Model file for the job. Use its own axes, mm. Coordinates: 2 decimals unless noted, no trailing zeros. Write each loop counter-clockwise with the first axis right and the second up, starting at its lowest first coordinate (ties: lowest second). Pieces come first, ordered by that corner, then holes. Notation, with made-up numbers: (36.25, 56.25) - (92.25, 56.25) arc R19 cw to (92.25, 84.25) - close; hole circle Ø6 at (51.5, 71.25). An arc over 180 degrees is marked (long way). Put each result on its own line as item: value. Start each with the question number.
1. Saw through at C-C, the plane z = -2.25. Write the cut outline in (x, y), plus the area to 3 significant figures.
2. Drill centre lines: L1, parallel to Z at x = 92, y = -12; L2, parallel to Y at x = 100, z = -7.25; L3, parallel to Z at x = 93.5, y = -10.25. Where is each one in solid material? Low to high. Write a range as from..to.
3. Saw through at B-B, the plane x = 99.75. Write the cut outline in (y, z).
4. Saw through at A-A, the plane y = -11.25. Write the cut outline in (x, z).
```python
from build123d import *

# Parameters (mm, degrees)
SKETCH032_W     = 16
SKETCH032_H     = 16
PAD017_DEPTH    = 28.8
POCKET015_DEPTH = 16
SKETCH115_W     = 1
SKETCH115_H     = 16
POCKET031_DEPTH = 30
PAD134_DEPTH    = 14


with BuildPart() as part:
    # Sketch032 (on Face52 of Binder013) → Pad017 (new body)
    with BuildSketch(Plane.XY.offset(-28.8)):
        with Locations((96, -8)):
            Rectangle(SKETCH032_W, SKETCH032_H)
    extrude(amount=PAD017_DEPTH)

    # Sketch033 (on Face2 of Pad017) → Pocket015 (cut)
    with BuildSketch(Plane.YZ.offset(104)):
        Polygon((-16, 0), (-16, -9.6), (0, 0), align=None)
    extrude(amount=-POCKET015_DEPTH, mode=Mode.SUBTRACT)

    # Sketch115 (on Face2 of Pocket015) → Pocket031 (cut)
    with BuildSketch(Plane(origin=(0, 0, -28.8), x_dir=(1, 0, 0), z_dir=(0, 0, -1))):
        with Locations((103.5, 8)):
            Rectangle(SKETCH115_W, SKETCH115_H)
        with Locations((88.5, 8)):
            Rectangle(SKETCH115_W, SKETCH115_H)
    extrude(amount=-POCKET031_DEPTH, mode=Mode.SUBTRACT)

    # Sketch134 (on Face3 of Pocket031) → Pad134 (join)
    with BuildSketch(Plane.YZ.offset(103)):
        Polygon((0, 0), (-3.2, 0), (-16, -7.68), (-16, -10.88), (-3.2, -3.2), (0, -3.2), align=None)
    extrude(amount=-PAD134_DEPTH)


solid = part.part
```
Final values:
1. outline: (89, -6.95) - (103, -6.95) - (103, 0) - (89, 0) - close
1. area: 97.3 mm²
2. L1: z = -28.8..-5.28
2. L2: y = -15.28..0
2. L3: z = -28.8..-4.23
3. outline: (-16, -28.8) - (0, -28.8) - (0, 0) - (-3.2, 0) - (-16, -7.68) - close
4. outline: (89, -28.8) - (103, -28.8) - (103, -4.83) - (89, -4.83) - close
